```python
from build123d import *

# Parameters (mm, degrees)
SKETCH_1_W          = 120
SKETCH_1_H          = 170
EXTRUDE_1_DEPTH     = 1.5
SKETCH_2_W          = 80
SKETCH_2_H          = 2
EXTRUDE_2_DEPTH     = 9
SKETCH_3_R          = 1.6
CUT_EXTRUDE_1_DEPTH = 9


with BuildPart() as part:
    # 草图1 → 凸台-拉伸1 (new body)
    with BuildSketch(Plane.XY):
        with Locations((60, -85)):
            Rectangle(SKETCH_1_W, SKETCH_1_H)
    extrude(amount=EXTRUDE_1_DEPTH)

    # 草图2 → 凸台-拉伸2 (add)
    with BuildSketch(Plane.XY.offset(1.5)):
        with Locations((40, -169)):
            Rectangle(SKETCH_2_W, SKETCH_2_H)
    extrude(amount=EXTRUDE_2_DEPTH)

    # 草图3 → 切除-拉伸1 (cut)
    with BuildSketch(Plane(origin=(0, -168, 0), x_dir=(1, 0, 0), z_dir=(0, 1, 0))):
        with Locations(Location((20, -6, 0), (0, 0, 270))):
            Circle(SKETCH_3_R)
        with Locations(Location((40, -6, 0), (0, 0, 270))):
            Circle(SKETCH_3_R)
        with Locations(Location((60, -6, 0), (0, 0, 270))):
            Circle(SKETCH_3_R)
    extrude(amount=-CUT_EXTRUDE_1_DEPTH, mode=Mode.SUBTRACT)


solid = part.part
```
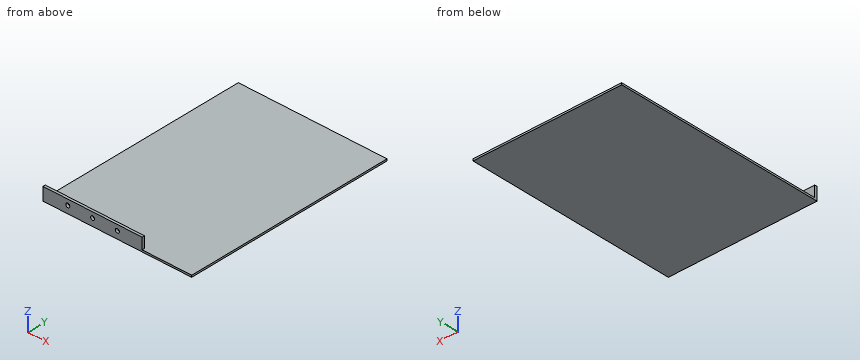
Read the model definition and answer for the solid it produces. Units are mm, in the model's axes. Give positions to 0.01 mm unless a question says otherwise; leave off trailing zeros. Write each loop counter-clockwise with the first axis right and the second up, starting at its lowest first coordinate (ties: lowest second). Pieces come first, ordered by that corner, then holes. Notation, with made-up numbers: (58.25, 74.5) -> (94.25, 74.5) arc R23 cw to (94.25, 83.5) -> close; hole circle Ø7 at (48, 38). An arc over 180 degrees is marked (long way). Answer as a JSON object with one key per item and string values.
1) Straight lines are drawn through the part: probe 1 along X at (y, z) = (-168.45, 6); probe 2 along Y at (x, z) = (70, 7.75); probe 3 along Z at (x, y) = (9, -83.5). For each, find the intervals that lie inside material, in ascending order. Write a range as from..to.
Findings below:
{"probe 1": "x = 0..18.4, 21.6..38.4, 41.6..58.4, 61.6..80", "probe 2": "y = -170..-168", "probe 3": "z = 0..1.5"}
2) Section D-D on x = 85.5 is taken. Write down the section's boundary in (y, z).
Findings below:
{"outline": "(-170, 0) -> (0, 0) -> (0, 1.5) -> (-170, 1.5) -> close"}
3) Section C-C on y = -16.5 is taken. Write down the section's boundary in (x, z), then the cut area to 3 significant figures.
Findings below:
{"outline": "(0, 0) -> (120, 0) -> (120, 1.5) -> (0, 1.5) -> close", "area": "180 mm^2"}
4) Section A-A on z = 6 is taken. Write down the section's boundary in (x, y), then the cut area to 3 significant figures.
Findings below:
{"outline": "(0, -170) -> (18.4, -170) -> (18.4, -168) -> (0, -168) -> close; (21.6, -170) -> (38.4, -170) -> (38.4, -168) -> (21.6, -168) -> close; (41.6, -170) -> (58.4, -170) -> (58.4, -168) -> (41.6, -168) -> close; (61.6, -170) -> (80, -170) -> (80, -168) -> (61.6, -168) -> close", "area": "141 mm^2"}
5) Flat-ended cylindrical pins translate along their axes: pin 1 Ø2 at (y, z) = (-169, 8) entering from +X; pin 2 Ø4.5 at (x, z) = (28, 6) entering from +Y; pin 3 Ø1.5 at (x, y) = (31.5, -39) entering from +Z. Find the tip coordinate at first contact, or state that the pin passes through.
Findings below:
{"pin 1": "stops at x = 80", "pin 2": "stops at y = -168", "pin 3": "stops at z = 1.5"}
6) Section B-B on x = 67 is taken. Write down the section's boundary in (y, z).
Findings below:
{"outline": "(-170, 0) -> (0, 0) -> (0, 1.5) -> (-168, 1.5) -> (-168, 10.5) -> (-170, 10.5) -> close"}
